from build123d import *

# Parameters (mm, degrees)
SKETCH_1_R          = 10
EXTRUDE_1_DEPTH     = 30
SKETCH_2_R          = 5
EXTRUDE_2_DEPTH     = 30
EXTRUDE_START       = 30
SKETCH_3_R          = 5
EXTRUDE_3_DEPTH     = 30
SKETCH_4_R          = 2
CUT_EXTRUDE_1_DEPTH = 20
CUT_EXTRUDE_START   = -20
SKETCH_5_R          = 2
CUT_EXTRUDE_2_DEPTH = 20


with BuildPart() as part:
    # 草图1 → 凸台-拉伸1 (new body)
    with BuildSketch(Plane(origin=(0, 0, 0), x_dir=(1, 0, 0), z_dir=(0, 1, 0))):
        with Locations(Location((0, 0, 0), (0, 0, 270))):
            Circle(SKETCH_1_R)
    extrude(amount=EXTRUDE_1_DEPTH)

    # 草图2 → 凸台-拉伸2 (add)
    with BuildSketch(Plane(origin=(0, 30, 0), x_dir=(1, 0, 0), z_dir=(0, 1, 0))):
        with Locations(Location((0, 0, 0), (0, 0, 270))):
            Circle(SKETCH_2_R)
    extrude(amount=EXTRUDE_2_DEPTH)

    # 草图3 → 凸台-拉伸3 (add)
    with BuildSketch(Plane(origin=(0, 0, 0), x_dir=(-1, 0, 0), z_dir=(0, -1, 0)).offset(EXTRUDE_START)):
        with Locations(Location((0, 0, 0), (0, 0, 270))):
            Circle(SKETCH_3_R)
    extrude(amount=-EXTRUDE_3_DEPTH)

    # 草图4 → 切除-拉伸1 (cut)
    with BuildSketch(Plane(origin=(0, 60, 0), x_dir=(1, 0, 0), z_dir=(0, 1, 0))):
        with Locations(Location((0, 0, 0), (0, 0, 270))):
            Circle(SKETCH_4_R)
    extrude(amount=-CUT_EXTRUDE_1_DEPTH, mode=Mode.SUBTRACT)

    # 草图5 → 切除-拉伸2 (cut)
    with BuildSketch(Plane(origin=(0, -30, 0), x_dir=(-1, 0, 0), z_dir=(0, -1, 0)).offset(CUT_EXTRUDE_START)):
        with Locations(Location((0, 0, 0), (0, 0, 270))):
            Circle(SKETCH_5_R)
    extrude(amount=CUT_EXTRUDE_2_DEPTH, mode=Mode.SUBTRACT)


solid = part.part
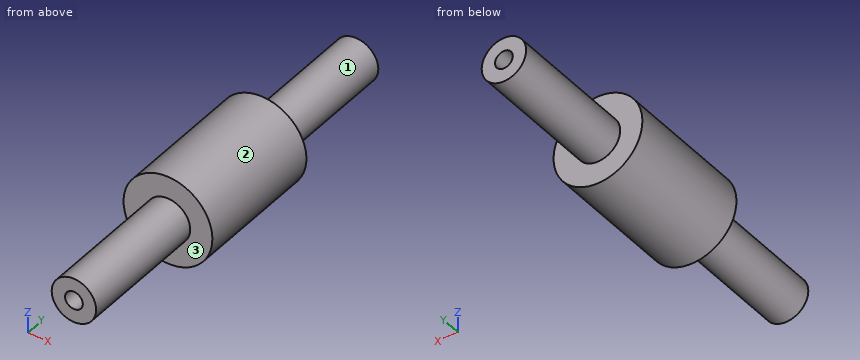
Design review of the part built by this model. Coordinates are the model's own, in mm. Face numbers are marked on the shaded views. A direction names the side the tool comes from. Round coordinates to 2 decimals unless told otherwise and drop trailing zeros. Loops run counter-clockwise (first coordinate to the right, second up) from the corner with the lowest first, then second, coordinate; pieces in that order, holes last. Notation, with made-up numbers: (-6.75, -31) - (45.25, -31) arc R25 cw to (45.25, -5) - close; hole circle Ø10 at (-35.5, -11). An arc over 180 degrees is marked (long way). One line per item, written item: value. Start each with the question number.
1) Consider section A-A on x = 0. Give the boundary of the cut face in (y, z).
2) Consider section C-C on y = -1.5. Give the boundary of the cut face in (x, z), then the cut area to 3 significant figures.
3) Consider section B-B on z = 0. Give the boundary of the cut face in (x, y).
4) For the marked faces 1, 2 and 3, list the 3-axis set-ups (+Z, -Z, +X, -X, +Y, -Y) from which the entire face can be reached by the end or side of a thin tool; tool diameter is ignored.
5) Consider section D-D on y = -18. Give the boundary of the cut face in (x, z), then the cut area to 3 significant figures.
6) Insertion check: pin 1 Ø1 at (y, z) = (25.5, -5.5) entering from -X; pin 2 Ø1 at (x, z) = (-6, -0.5) entering from +Y; pin 3 Ø1.5 at (y, z) = (-17.5, 1.5) entering from +X. Each pin has a flat end and moves straight along its axis. Give the tip position at first contact, or say it passes through.
7) To check wall thickness, follow L1, parallel to X at y = 45, z = 0; L2, parallel to Y at x = 2.5, z = 9; L3, parallel to Y at x = -0.5, z = -1. State the ranges of each line that lie inside material, in increasing order. Write a range as from..to.
Reported:
1. outline: (-30, -5) - (0, -5) - (0, -10) - (30, -10) - (30, -5) - (60, -5) - (60, -2) - (40, -2) - (40, 2) - (60, 2) - (60, 5) - (30, 5) - (30, 10) - (0, 10) - (0, 5) - (-30, 5) - (-30, 2) - (-10, 2) - (-10, -2) - (-30, -2) - close
2. outline: circle Ø10 at (0, 0)
2. area: 78.5 mm^2
3. outline: (-10, 0) - (-5, 0) - (-5, -30) - (-2, -30) - (-2, -10) - (2, -10) - (2, -30) - (5, -30) - (5, 0) - (10, 0) - (10, 30) - (5, 30) - (5, 60) - (2, 60) - (2, 40) - (-2, 40) - (-2, 60) - (-5, 60) - (-5, 30) - (-10, 30) - close
4. face 1: +Y
4. face 2: +Y, -Y
4. face 3: -Y
5. outline: circle Ø10 at (0, 0); hole circle Ø4 at (0, 0)
5. area: 66.0 mm^2
6. pin 1: stops at x = -8.66
6. pin 2: stops at y = 30
6. pin 3: stops at x = 4.94
7. L1: x = -5..-2, 2..5
7. L2: y = 0..30
7. L3: y = -10..40
